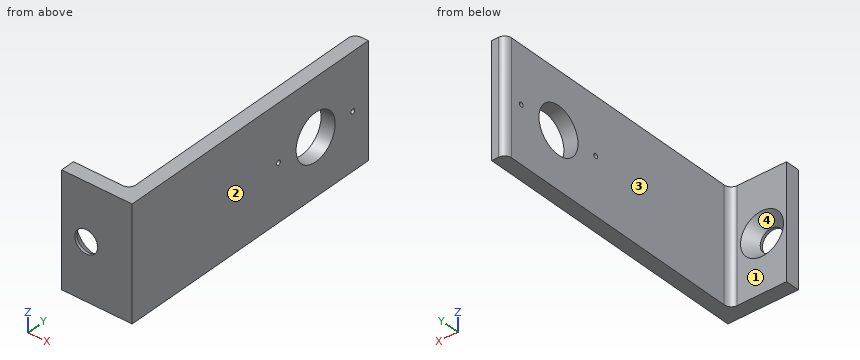
from build123d import *

# Parameters (mm, degrees)
BOSS_EXTRUDE1_DEPTH = 25.4
SKETCH3_R           = 4.765
CUT_EXTRUDE1_DEPTH  = 128
SKETCH4_R           = 10.5
CUT_EXTRUDE2_DEPTH  = 12.7
SKETCH5_R           = 1.04
CUT_EXTRUDE3_DEPTH  = 10


with BuildPart() as part:
    # Sketch2 → Boss-Extrude1 (new body, symmetric)
    with BuildSketch(Plane.XY):
        with BuildLine():
            Line((-15.875, 0), (15.875, 0))
            Line((15.875, 0), (15.875, 127))
            Line((15.875, 127), (12.7, 127))
            ThreePointArc((12.7, 127), (10.45493597, 126.07006403), (9.525, 123.825))
            Line((9.525, 123.825), (9.525, 9.525))
            ThreePointArc((9.525, 9.525), (8.59506403, 7.27993597), (6.35, 6.35))
            Line((6.35, 6.35), (-15.875, 6.35))
            Line((-15.875, 6.35), (-15.875, 0))
        make_face()
    extrude(amount=BOSS_EXTRUDE1_DEPTH, both=True)

    # Sketch3 → Cut-Extrude1 (cut, through all)
    with BuildSketch(Plane.XZ):
        with Locations((-4.826, 0)):
            Circle(SKETCH3_R)
    extrude(amount=-CUT_EXTRUDE1_DEPTH, mode=Mode.SUBTRACT)

    # Sketch4 → Cut-Extrude2 (cut)
    with BuildSketch(Plane(origin=(15.875, 0, 0), x_dir=(0, 0, -1), z_dir=(1, 0, 0))):
        with Locations((0, 98.65)):
            Circle(SKETCH4_R)
    extrude(amount=-CUT_EXTRUDE2_DEPTH, mode=Mode.SUBTRACT)

    # Sketch5 → Cut-Extrude3 (cut)
    with BuildSketch(Plane(origin=(15.875, 0, 0), x_dir=(0, 0, -1), z_dir=(1, 0, 0))):
        with Locations((0, 78.65)):
            Circle(SKETCH5_R)
        with Locations((0, 118.65)):
            Circle(SKETCH5_R)
    extrude(amount=-CUT_EXTRUDE3_DEPTH, mode=Mode.SUBTRACT)

    # Sketch7 → CSK for 3/8 Flat Head Machine Screw1 (revolve, cut)
    with BuildSketch(Plane(origin=(-4.826, 6.35, 0), x_dir=(0, 0, 1), z_dir=(1, 0, 0))):
        Polygon((0, 0), (0, 6.35), (5.15874, 6.35), (5.15874, 5.198123707), (9.6774, 0), align=None)
    revolve(axis=Axis((-4.826, 12.7, 0), (0, -1, 0)), mode=Mode.SUBTRACT)


solid = part.part
Build history of the part. All positions in model axes, mm. Face numbers are marked on the shaded views. Round coordinates to 2 decimals unless told otherwise and drop trailing zeros. Loops run counter-clockwise (first coordinate to the right, second up) from the corner with the lowest first, then second, coordinate; pieces in that order, holes last. Notation, with made-up numbers: (-32, -26.5) -> (-11, -26.5) arc R28 cw to (-11, 6.5) -> close; hole circle Ø6 at (58.25, -33.75). An arc over 180 degrees is marked (long way). Use CSV: the item, a comma, the result in double quotes. Start each with the question number.
Q1. Saw through at B-B on z = -21.5. Give the cut face in (x, y) (3 decimals), and give its area (3 significant figures).
Q2. Saw through at C-C on y = 62. Give the cut face in (x, z) (3 decimals).
Q3. Drill centre lines: L1, parallel to X at y = 0.65, z = 0 (3 decimals); L2, parallel to Y at x = 13, z = 0; L3, parallel to Y at x = 11.5, z = 0. Where is each one in solid material? Low to high.
Q4. Flat gauge pins, fed straight in: pin 1 Ø1 at (x, z) = (-9.5, 16) entering from +Y; pin 2 Ø15 at (y, z) = (93, -12) entering from -X (3 decimals). Where does each tip first touch, or does it go through?
Q5. Mould opens along X. For the marked faces 1, 2, 3 and 4 say: +X half, -X half, draft (parallel to the pull), parting line (faces both ways), or undercut.
Q6. Saw through at A-A on y = 98.65. Give the cut face in (x, z) (3 decimals), and give its area (3 significant figures).
Solutions:
1,outline,"(-15.875, 0) -> (15.875, 0) -> (15.875, 127) -> (12.7, 127) arc R3.175 ccw to (9.525, 123.825) -> (9.525, 9.525) arc R3.175 cw to (6.35, 6.35) -> (-15.875, 6.35) -> close"
1,area,"968 mm^2"
2,outline,"(9.525, -25.4) -> (15.875, -25.4) -> (15.875, 25.4) -> (9.525, 25.4) -> close"
3,L1,"x = -15.875 to -9.985, 0.333 to 15.875"
3,L2,"y = 0 to 77.61, 79.69 to 88.15, 109.15 to 117.61, 119.69 to 127"
3,L3,"y = 0 to 77.61, 79.69 to 88.15, 109.15 to 117.61, 119.69 to 126.76"
4,pin 1,"stops at y = 6.35"
4,pin 2,"stops at x = 9.525"
5,face 1,"draft"
5,face 2,"+X half"
5,face 3,"-X half"
5,face 4,"undercut"
6,outline,"(9.525, -25.4) -> (15.875, -25.4) -> (15.875, -10.5) -> (9.525, -10.5) -> close; (9.525, 10.5) -> (15.875, 10.5) -> (15.875, 25.4) -> (9.525, 25.4) -> close"
6,area,"189 mm^2"
